```python
from build123d import *

# Parameters (mm, degrees)
SKETCH1_W           = 20.828
SKETCH1_H           = 20.066
BOSS_EXTRUDE1_DEPTH = 25.4
CAVITY1_START       = 4.562
CAVITY1_OUTLINE_W   = 8.89
CAVITY1_OUTLINE_H   = 14.9
CAVITY1_DEPTH       = 11.938
CAVITY1_START_2     = 9.031
CAVITY1_2_OUTLINE_W = 2.11
CAVITY1_2_OUTLINE_H = 14.9
CAVITY1_2_DEPTH     = 3


# Read off the part's stored shape, not the designer's step: Cavity1
with BuildPart() as part:
    # Sketch1 → Boss-Extrude1 (new body)
    with BuildSketch(Plane.XY):
        with Locations((10.414, 10.033)):
            Rectangle(SKETCH1_W, SKETCH1_H)
    extrude(amount=-BOSS_EXTRUDE1_DEPTH)

    # Cavity1 outline → Cavity1 (cut)
    with BuildSketch(Plane.YZ.offset(CAVITY1_START)):
        with Locations((9.945, -7.45)):
            Rectangle(CAVITY1_OUTLINE_W, CAVITY1_OUTLINE_H)
    extrude(amount=CAVITY1_DEPTH, mode=Mode.SUBTRACT)

    # Cavity1 2 outline → Cavity1 2 (cut)
    with BuildSketch(Plane.YZ.offset(CAVITY1_START_2)):
        with Locations((4.445, -7.45)):
            Rectangle(CAVITY1_2_OUTLINE_W, CAVITY1_2_OUTLINE_H)
    extrude(amount=CAVITY1_2_DEPTH, mode=Mode.SUBTRACT)


solid = part.part
```
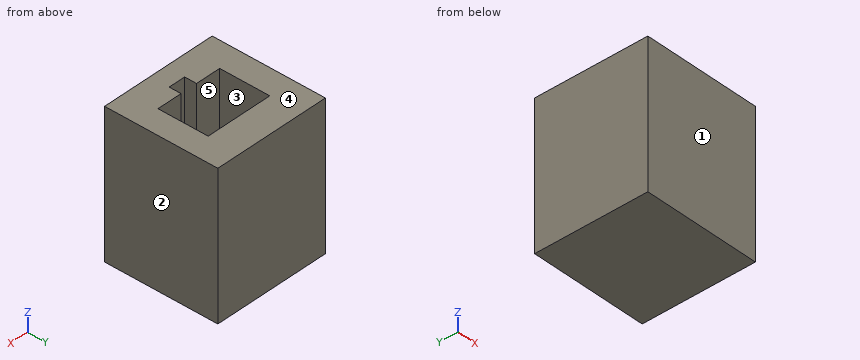
Verification items for the finished model (mm, model axes). Face numbers are marked on the shaded views. A direction names the side the tool comes from. Round coordinates to 2 decimals unless told otherwise and drop trailing zeros. Order: outer loops, then holes, each group sorted by start corner. A loop starts at its lowest first (then second) coordinate and runs counter-clockwise, first axis right, second up.
1) Cross-section at B-B, the plane x = 10. Record the cut outline in (y, z), plus the area to 3 significant figures.
Geometry says:
outline: (0, -25.4) - (20.07, -25.4) - (20.07, 0) - (14.39, 0) - (14.39, -14.9) - (3.39, -14.9) - (3.39, 0) - (0, 0) - close
area: 346 mm2
2) Depth check by flat-ended pin: pin 1 (8 mm diameter, centred on x = 16, y = 4.5, fed in from +Z); pin 2 (3.5 mm diameter, centred on x = 12.5, y = 11, fed in from +Z). Enter the tip coordinate at first touch or a pass-through.
Geometry says:
pin 1: stops at z = 0
pin 2: stops at z = -14.9
3) Material ranges on line 1 (Y direction, x = 13.25, z = -6); line 2 (Y direction, x = 11, z = -10.75); line 3 (X direction, y = 8.5, z = -6), recorded low to high.
Geometry says:
line 1: y = 0 to 5.5, 14.39 to 20.07
line 2: y = 0 to 3.39, 14.39 to 20.07
line 3: x = 0 to 4.56, 16.5 to 20.83
4) Tool access check on the marked faces 4 and 5. Record the directions out of +Z, -Z, +X, -X, +Y, -Y that give a thin tool (end or side, any length) a straight path to the whole face; none if there is none.
Geometry says:
face 4: +Z, +X, -X, +Y, -Y
face 5: +Z
5) Cross-section at C-C, the plane y = 13. Record the cut outline in (x, z).
Geometry says:
outline: (0, -25.4) - (20.83, -25.4) - (20.83, 0) - (16.5, 0) - (16.5, -14.9) - (4.56, -14.9) - (4.56, 0) - (0, 0) - close
6) Cross-section at A-A, the plane z = -9.5. Record the cut outline in (x, y).
Geometry says:
outline: (0, 0) - (20.83, 0) - (20.83, 20.07) - (0, 20.07) - close; hole (4.56, 5.5) - (9.03, 5.5) - (9.03, 3.39) - (12.03, 3.39) - (12.03, 5.5) - (16.5, 5.5) - (16.5, 14.39) - (4.56, 14.39) - close
7) Draft check along X on the marked faces 1, 2 and 3. Enter one of: +X half, -X half, draft (parallel to the pull), parting line (faces both ways), or undercut.
Geometry says:
face 1: draft
face 2: +X half
face 3: undercut
